The model under review builds one solid part; all positions refer to its coordinate system, in mm. Round coordinates to 2 decimals unless told otherwise and drop trailing zeros. Loops run counter-clockwise (first coordinate to the right, second up) from the corner with the lowest first, then second, coordinate; pieces in that order, holes last. Notation, with made-up numbers: M 43,28 L 102,28 A18 ccw 102,40 Z; hole C 77.5,2 d7. An arc over 180 degrees is marked long. Answer as a JSON object with one key per item and string values. Group by question number.
Item 1: To check wall thickness, follow line 1 (Y direction, x = 75, z = 0.7); line 2 (Y direction, x = 15, z = 0.7); line 3 (X direction, y = 11, z = 1.2). State the ranges of each line that lie inside material, in increasing order.
Item 2: Consider section D-D (y = 20). Give the boundary of the cut face in (x, z), and give its area (3 significant figures).
Item 3: Consider section A-A (y = 60). Give the boundary of the cut face in (x, z), and give its area (3 significant figures).
Item 4: Consider section C-C (z = 1.35). Give the boundary of the cut face in (x, y).
Item 5: The part is to be moulded in two halves that separate along Y. For faces 1 (the face through (73.568, 70.906, 1.014)), 2 (the face through (74, 80, 0)), say which applies: +Y half, -Y half, draft (parallel to the pull), parting line (faces both ways), or undercut.
Item 6: Consider section B-B (x = 135). Give the boundary of the cut face in (y, z), and give its area (3 significant figures).
Autodesk Inventor part; units mm, degrees
ref_plane "YZ Plane" through (0, 0, 0) normal (1, 0, 0) x (0, 1, 0)
ref_plane "XZ Plane" through (0, 0, 0) normal (0, 1, 0) x (-1, 0, 0)
ref_plane "XY Plane" through (0, 0, 0) normal (0, 0, 1) x (1, 0, 0)
sketch "Sketch1" plane through (0, 0, 0) normal (0, 0, 1) x (1, 0, 0)
  line L0 (0, 0) -> (150, 0)
  line L1 (150, 0) -> (150, 157)
  line L2 (150, 157) -> (0, 157)
  line L3 (0, 157) -> (0, 0)
  dimension "d0" = 157
  dimension "d1" = 150
extrude "Plate1" add sketch "Sketch1" along normal blind 2
sketch "Sketch2" plane through (0, 0, 2) normal (0, 0, 1) x (1, 0, 0)
  line L0 (0, 0) -> (0, 157)
  line L1 (0, 157) -> (150, 157)
  circle A0 centre (75, 60) radius 11
  line L2 (150, 0) -> (0, 0)
  line L3 (150, 157) -> (150, 0)
  circle A1 centre (15, 10) radius 2.5
  circle A2 centre (15, 20) radius 2.5
  line L4 (75, 0) -> (75, 157) construction
  circle A3 centre (135, 10) radius 2.5
  circle A4 centre (135, 20) radius 2.5
  circle A5 centre (75, 93) radius 4.5
  point P0 (0, 78.5)
  dimension "d3" = 22
  dimension "d6" = 5
  dimension "d7" = 5
  dimension "d8" = 15
  dimension "d9" = 10
  dimension "d10" = 10
  dimension "d11" = 9
  dimension "d12" = 33
  dimension "d13" = 60
extrude "Extrusion1" cut sketch "Sketch2" against normal through all contours A0 | A1 | A2 | A3 | A4 | A5
equation "\"BendRadius\" = Thickness"
equation "\"BendReliefWidth\" = Thickness"
equation "\"BendReliefDepth\" = 0.5 * Thickness"
equation "\"CornerReliefSize\" = 4 * Thickness"
equation "\"MinimumRemnant\" = 2 * Thickness"
equation "\"TransitionRadius\" = BendRadius"
equation "\"JacobiRadiusSize\" = BendRadius"
equation "\"GapSize\" = Thickness"
equation "\"d2\" = BendRadius"
properties part number "SensorPlatta"
Geometry results:
{
 "1": {"line 1": "y = 0 to 49, 71 to 88.5, 97.5 to 157", "line 2": "y = 0 to 7.5, 12.5 to 17.5, 22.5 to 157", "line 3": "x = 0 to 12.71, 17.29 to 132.71, 137.29 to 150"},
 "2": {"outline": "M 0,0 L 12.5,0 L 12.5,2 L 0,2 Z; M 17.5,0 L 132.5,0 L 132.5,2 L 17.5,2 Z; M 137.5,0 L 150,0 L 150,2 L 137.5,2 Z", "area": "280 mm^2"},
 "3": {"outline": "M 0,0 L 64,0 L 64,2 L 0,2 Z; M 86,0 L 150,0 L 150,2 L 86,2 Z", "area": "256 mm^2"},
 "4": {"outline": "M 0,0 L 150,0 L 150,157 L 0,157 Z; hole C 15,10 d5; hole C 15,20 d5; hole C 75,60 d22; hole C 75,93 d9; hole C 135,10 d5; hole C 135,20 d5"},
 "5": {"face 1": "undercut", "face 2": "draft"},
 "6": {"outline": "M 0,0 L 7.5,0 L 7.5,2 L 0,2 Z; M 12.5,0 L 17.5,0 L 17.5,2 L 12.5,2 Z; M 22.5,0 L 157,0 L 157,2 L 22.5,2 Z", "area": "294 mm^2"}
}
